```python
from build123d import *

# Parameters (mm, degrees)
SKETCH_1_W      = 350
SKETCH_1_H      = 350
SKETCH_1_R      = 1.5
EXTRUDE_1_DEPTH = 3
FILLET_1_R      = 10


with BuildPart() as part:
    # Sketch 1 → Extrude 1 (new body)
    with BuildSketch(Plane.XY):
        with Locations((175, 175)):
            Rectangle(SKETCH_1_W, SKETCH_1_H)
        with Locations((10, 20)):
            Circle(SKETCH_1_R, mode=Mode.SUBTRACT)
        with Locations((40, 20)):
            Circle(SKETCH_1_R, mode=Mode.SUBTRACT)
        with Locations((70, 20)):
            Circle(SKETCH_1_R, mode=Mode.SUBTRACT)
        with Locations((100, 20)):
            Circle(SKETCH_1_R, mode=Mode.SUBTRACT)
        with Locations((130, 20)):
            Circle(SKETCH_1_R, mode=Mode.SUBTRACT)
        with Locations((160, 20)):
            Circle(SKETCH_1_R, mode=Mode.SUBTRACT)
        with Locations((190, 20)):
            Circle(SKETCH_1_R, mode=Mode.SUBTRACT)
        with Locations((220, 20)):
            Circle(SKETCH_1_R, mode=Mode.SUBTRACT)
        with Locations((250, 20)):
            Circle(SKETCH_1_R, mode=Mode.SUBTRACT)
        with Locations((280, 20)):
            Circle(SKETCH_1_R, mode=Mode.SUBTRACT)
        with Locations((310, 20)):
            Circle(SKETCH_1_R, mode=Mode.SUBTRACT)
        with Locations((340, 20)):
            Circle(SKETCH_1_R, mode=Mode.SUBTRACT)
        with Locations((40, 40)):
            Circle(SKETCH_1_R, mode=Mode.SUBTRACT)
        with Locations((70, 40)):
            Circle(SKETCH_1_R, mode=Mode.SUBTRACT)
        with Locations((100, 40)):
            Circle(SKETCH_1_R, mode=Mode.SUBTRACT)
        with Locations((130, 40)):
            Circle(SKETCH_1_R, mode=Mode.SUBTRACT)
        with Locations((160, 40)):
            Circle(SKETCH_1_R, mode=Mode.SUBTRACT)
        with Locations((190, 40)):
            Circle(SKETCH_1_R, mode=Mode.SUBTRACT)
        with Locations((220, 40)):
            Circle(SKETCH_1_R, mode=Mode.SUBTRACT)
        with Locations((250, 40)):
            Circle(SKETCH_1_R, mode=Mode.SUBTRACT)
        with Locations((280, 40)):
            Circle(SKETCH_1_R, mode=Mode.SUBTRACT)
        with Locations((310, 40)):
            Circle(SKETCH_1_R, mode=Mode.SUBTRACT)
        with Locations((340, 40)):
            Circle(SKETCH_1_R, mode=Mode.SUBTRACT)
        with Locations((10, 40)):
            Circle(SKETCH_1_R, mode=Mode.SUBTRACT)
        with BuildLine():
            Line((25, 321.5), (125, 321.5))
            ThreePointArc((125, 321.5), (126.5, 320), (125, 318.5))
            Line((125, 318.5), (25, 318.5))
            ThreePointArc((25, 318.5), (23.5, 320), (25, 321.5))
        make_face(mode=Mode.SUBTRACT)
        with BuildLine():
            Line((25, 247.5), (125, 247.5))
            ThreePointArc((125, 247.5), (126.5, 246), (125, 244.5))
            Line((125, 244.5), (25, 244.5))
            ThreePointArc((25, 244.5), (23.5, 246), (25, 247.5))
        make_face(mode=Mode.SUBTRACT)
        with BuildLine():
            Line((325, 247.5), (225, 247.5))
            ThreePointArc((225, 247.5), (223.5, 246), (225, 244.5))
            Line((225, 244.5), (325, 244.5))
            ThreePointArc((325, 244.5), (326.5, 246), (325, 247.5))
        make_face(mode=Mode.SUBTRACT)
        with BuildLine():
            Line((325, 321.5), (225, 321.5))
            ThreePointArc((225, 321.5), (223.5, 320), (225, 318.5))
            Line((225, 318.5), (325, 318.5))
            ThreePointArc((325, 318.5), (326.5, 320), (325, 321.5))
        make_face(mode=Mode.SUBTRACT)
        with BuildLine():
            Line((176.5, 210), (176.5, 103.615907309))
            ThreePointArc((176.5, 103.615907309), (175, 102.115907309), (173.5, 103.615907309))
            Line((173.5, 103.615907309), (173.5, 210))
            ThreePointArc((173.5, 210), (175, 211.5), (176.5, 210))
        make_face(mode=Mode.SUBTRACT)
        with BuildLine():
            Line((186.5, 210), (186.5, 103.615907309))
            ThreePointArc((186.5, 103.615907309), (185, 102.115907309), (183.5, 103.615907309))
            Line((183.5, 103.615907309), (183.5, 210))
            ThreePointArc((183.5, 210), (185, 211.5), (186.5, 210))
        make_face(mode=Mode.SUBTRACT)
        with BuildLine():
            Line((163.5, 210), (163.5, 103.615907309))
            ThreePointArc((163.5, 103.615907309), (165, 102.115907309), (166.5, 103.615907309))
            Line((166.5, 103.615907309), (166.5, 210))
            ThreePointArc((166.5, 210), (165, 211.5), (163.5, 210))
        make_face(mode=Mode.SUBTRACT)
    extrude(amount=EXTRUDE_1_DEPTH)

    # Fillet 1
    fillet_1_edges = [part.edges().sort_by_distance(p)[0] for p in [
        (350, 350, 1.5),
        (350, 0, 1.5),
        (0, 0, 1.5),
        (0, 350, 1.5),
    ]]
    fillet(fillet_1_edges, radius=FILLET_1_R)


solid = part.part
```
Geometry: final body of the model. Coordinates: model frame, mm. Round coordinates to 2 decimals unless told otherwise and drop trailing zeros. Loops run counter-clockwise (first coordinate to the right, second up) from the corner with the lowest first, then second, coordinate; pieces in that order, holes last. Notation, with made-up numbers: (64, 81.5) -> (92, 81.5) arc R22 ccw to (92, 112.5) -> close; hole circle Ø6 at (-12, -32). An arc over 180 degrees is marked (long way). Use one line per item in the form item = value.
Item 1: Material intervals for probe 1 along Y at (x, z) = (286.5, 2); probe 2 along Y at (x, z) = (160, 1.8); probe 3 along X at (y, z) = (184.5, 1.85), sorted ascending.
Evaluation:
probe_1 = 0 to 244.5, 247.5 to 318.5, 321.5 to 350
probe_2 = 0 to 18.5, 21.5 to 38.5, 41.5 to 350
probe_3 = 0 to 163.5, 166.5 to 173.5, 176.5 to 183.5, 186.5 to 350
Item 2: Cut plane B-B on z = 0.9. Give the number of separate pieces and of enclosed holes in the cut face, then the cut area to 3 significant figures.
Evaluation:
separate_pieces = 1
enclosed_holes = 31
area = 120,000 mm2
Item 3: Cut plane A-A on x = 316. Output: boundary loops of the cut face in (y, z).
Evaluation:
outline = (0, 0) -> (244.5, 0) -> (244.5, 3) -> (0, 3) -> close; (247.5, 0) -> (318.5, 0) -> (318.5, 3) -> (247.5, 3) -> close; (321.5, 0) -> (350, 0) -> (350, 3) -> (321.5, 3) -> close
